Source: CAD feature listing. Evaluate the final solid. Frame: model axes, mm. A direction names the side the tool comes from. Give positions to 0.01 mm unless a question says otherwise; leave off trailing zeros. Write each loop counter-clockwise with the first axis right and the second up, starting at its lowest first coordinate (ties: lowest second). Pieces come first, ordered by that corner, then holes.
```python
from build123d import *

# Parameters (mm, degrees)
F0_W           = 1524
F0_H           = 1016
F0_R           = 38.1
F1_DEPTH       = 101.6
F5_D           = 22
F5_CBORE_D     = 31.5
F5_CBORE_DEPTH = 20


with BuildPart() as f1:
    # F0 (on Front) → F1 (new body)
    with BuildSketch(Plane.XZ):
        with Locations((21.7913445085, 50.0460547454)):
            Rectangle(F0_W, F0_H)
        with Locations((-486.2086554915, -330.9539452546)):
            Circle(F0_R, mode=Mode.SUBTRACT)
        with Locations((529.7913445085, -330.9539452546)):
            Circle(F0_R, mode=Mode.SUBTRACT)
        with Locations((-486.2086554915, 431.0460547454)):
            Circle(F0_R, mode=Mode.SUBTRACT)
        with Locations((529.7913445085, 431.0460547454)):
            Circle(F0_R, mode=Mode.SUBTRACT)
    extrude(amount=F1_DEPTH)

    # F2 (on Top) → F3 (revolve)
    with BuildSketch(Plane.XY):
        Polygon((50.8, 508), (50.8, 0), (254, 0), (152.4, 508), align=None)
    revolve(axis=Axis((0, 140.2586251497, 0), (0, 1, 0)))

    # F5 (through all)
    with Locations(Plane.XZ.offset(101.6)):
        with Locations((0, 380.2460547454)):
            CounterBoreHole(F5_D / 2, F5_CBORE_D / 2, F5_CBORE_DEPTH)


solid = f1.part
```
1. Cut plane D-D, the plane x = 298. Return the cut outline in (y, z), then the cut area to 3 significant figures.
2. Mould query, pull axis Z, two halves, no side actions, for faces 1 (the flat face through (11, -50, 558.046)), 2 (the flat face through (11, -101.6, 57)), 3 (the flat face through (-1, 0, 1)). Classes: +Z half, -Z half, draft (parallel to the pull), parting line (faces both ways), or undercut.
3. Cut plane B-B, the plane y = 184. Return the cut outline in (x, z).
4. Line query: L1, parallel to Y at x = 330, z = 402.5; L2, parallel to Z at x = 4, y = 280.5; L3, parallel to X at y = 314, z = 0. Output: solid intervals per line, ascending.
5. Cut plane C-C, the plane z = 0. Return the cut outline in (x, y), then the cut area to 3 significant figures.
6. Contact query for flat-ended pins moving along their axis: P1, Ø1.5, axis at x = 195, y = 300, coming from the -Z side; P2, Ø1.5, axis at x = 161.5, y = 317, coming from the +Z side; P3, Ø25, axis at x = 0, z = 380.25, coming from the -Y side; P4, Ø8, axis at x = -346, z = 226.5, coming from the +Y side. Output: stop coordinate, or through.
7. Access query for faces 4 (the cylindrical face through (-451.014, -50.089, -345.546)), 5 (the flat face through (3, -81.6, 391)), 6 (the cylindrical face through (-11.012, 250.444, 49.592)). Directions: +Z, -Z, +X, -X, +Y, -Y. A direction counts if a zero-diameter tool reaches every point of the face in a straight line with its end or side. Return the directions, or none.
8. Cut plane A-A, the plane z = -346.5. Return the cut outline in (x, y).
Response values:
1. outline: (-101.6, -457.95) - (0, -457.95) - (0, 558.05) - (-101.6, 558.05) - close
1. area: 103,000 mm2
2. face 1: +Z half
2. face 2: draft
2. face 3: undercut
3. outline: circle Ø434.4 at (0, 0); hole circle Ø101.6 at (0, 0)
4. L1: y = -101.6 to 0
4. L2: z = -197.86 to -50.64, 50.64 to 197.86
4. L3: x = -191.2 to -50.8, 50.8 to 191.2
5. outline: (-740.21, -101.6) - (783.79, -101.6) - (783.79, 0) - (254, 0) - (152.4, 508) - (50.8, 508) - (50.8, 0) - (-50.8, 0) - (-50.8, 508) - (-152.4, 508) - (-254, 0) - (-740.21, 0) - close
5. area: 310,000 mm2
6. P1: passes through
6. P2: stops at z = 102.44
6. P3: stops at y = -81.6
6. P4: stops at y = 0
7. face 4: +Y, -Y
7. face 5: -Y
7. face 6: +Y
8. outline: (-740.21, -101.6) - (-520.99, -101.6) - (-520.99, 0) - (-740.21, 0) - close; (-451.42, -101.6) - (495.01, -101.6) - (495.01, 0) - (-451.42, 0) - close; (564.58, -101.6) - (783.79, -101.6) - (783.79, 0) - (564.58, 0) - close
